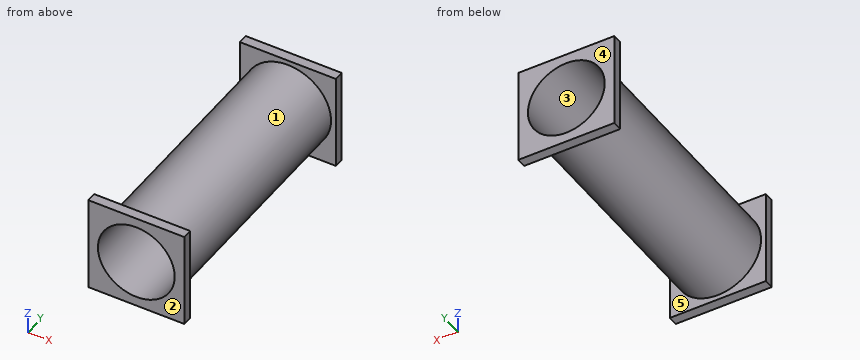
```python
from build123d import *

# Parameters (mm, degrees)
SKETCH1_W           = 20
SKETCH1_H           = 20
SKETCH1_R           = 8
BOSS_EXTRUDE1_DEPTH = 2
SKETCH2_R           = 9
SKETCH2_R_2         = 8
BOSS_EXTRUDE3_DEPTH = 50
SKETCH3_W           = 20
SKETCH3_H           = 20
SKETCH3_R           = 8
BOSS_EXTRUDE5_DEPTH = 2


with BuildPart() as part:
    # Sketch1 → Boss-Extrude1 (new body)
    with BuildSketch(Plane(origin=(0, 0, 0), x_dir=(1, 0, 0), z_dir=(0, 1, 0))):
        with Locations((-10, 10)):
            Rectangle(SKETCH1_W, SKETCH1_H)
        with Locations(Location((-10, 10, 0), (0, 0, 270))):
            Circle(SKETCH1_R, mode=Mode.SUBTRACT)
    extrude(amount=BOSS_EXTRUDE1_DEPTH)

    # Sketch2 → Boss-Extrude3 (add)
    with BuildSketch(Plane(origin=(0, 2, 0), x_dir=(1, 0, 0), z_dir=(0, 1, 0))):
        with Locations(Location((-10, 10, 0), (0, 0, 270))):
            Circle(SKETCH2_R)
        with Locations(Location((-10, 10, 0), (0, 0, 270))):
            Circle(SKETCH2_R_2, mode=Mode.SUBTRACT)
    extrude(amount=BOSS_EXTRUDE3_DEPTH)

    # Sketch3 → Boss-Extrude5 (add)
    with BuildSketch(Plane(origin=(0, 52, 0), x_dir=(1, 0, 0), z_dir=(0, 1, 0))):
        with Locations((-10, 10)):
            Rectangle(SKETCH3_W, SKETCH3_H)
        with Locations(Location((-10, 10, 0), (0, 0, 270))):
            Circle(SKETCH3_R, mode=Mode.SUBTRACT)
    extrude(amount=BOSS_EXTRUDE5_DEPTH)


solid = part.part
```
Geometry check sheet. Reference: the model listing, model coordinates, mm. Face numbers are marked on the shaded views. A direction names the side the tool comes from. Round coordinates to 2 decimals unless told otherwise and drop trailing zeros. Order: outer loops, then holes, each group sorted by start corner. A loop starts at its lowest first (then second) coordinate and runs counter-clockwise, first axis right, second up. Notation, with made-up numbers: M 82.25,-30 L 113.25,-30 A18 cw 113.25,-16 Z; hole C 48,76.5 d6. An arc over 180 degrees is marked long. Write item = value, one per line.
Q1. Scan lines: line 1 (Y direction, x = -15.75, z = -18.75); line 2 (X direction, y = 37.5, z = -10); line 3 (X direction, y = 28, z = -15.25). Record each from-to range of solid material in increasing order.
Answer block:
line_1 = 0 to 2, 52 to 54
line_2 = -19 to -18, -2 to -1
line_3 = -17.31 to -16.04, -3.96 to -2.69
Q2. Section check C-C (y = 13.5). Enter the section's corners in (x, z), plus the area to 3 significant figures.
Answer block:
outline = C -10,-10 d18; hole C -10,-10 d16
area = 53.4 mm^2
Q3. Depth check by flat-ended pin: pin 1 Ø8 at (x, y) = (-8, 47) entering from +Z; pin 2 Ø9.5 at (x, z) = (-10, -10) entering from +Y; pin 3 Ø1.5 at (x, y) = (-9, 29) entering from -Z; pin 4 Ø3 at (x, y) = (-14, 32) entering from -Z. Enter the tip coordinate at first touch or a pass-through.
Answer block:
pin_1 = -1
pin_2 = through
pin_3 = -19
pin_4 = -18.65
Q4. Set-up check for the marked faces 4 and 5: record each of +Z, -Z, +X, -X, +Y, -Y from which the full face is reachable in a straight line by a thin tool's end or side.
Answer block:
face_4 = +Z, -Z, +X, -X, +Y
face_5 = none
Q5. Release check for a two-part mould opening along X. For the marked faces 1, 2 and 3 record: released by +X, released by -X, zero draft, split by the parting line, or undercut.
Answer block:
face_1 = split by the parting line
face_2 = zero draft
face_3 = undercut
Q6. Section check B-B (z = -10). Enter the section's corners in (x, y), plus the area to 3 significant figures.
Answer block:
outline = M -20,0 L -18,0 L -18,54 L -20,54 L -20,52 L -19,52 L -19,2 L -20,2 Z; M -2,0 L 0,0 L 0,2 L -1,2 L -1,52 L 0,52 L 0,54 L -2,54 Z
area = 116 mm^2
Q7. Section check A-A (x = -10). Enter the section's corners in (y, z), plus the area to 3 significant figures.
Answer block:
outline = M 0,-20 L 2,-20 L 2,-19 L 52,-19 L 52,-20 L 54,-20 L 54,-18 L 0,-18 Z; M 0,-2 L 54,-2 L 54,0 L 52,0 L 52,-1 L 2,-1 L 2,0 L 0,0 Z
area = 116 mm^2
